The model under review builds one solid part; all positions refer to its coordinate system, in mm. Face numbers are marked on the shaded views. A direction names the side the tool comes from. Round coordinates to 2 decimals unless told otherwise and drop trailing zeros. Order: outer loops, then holes, each group sorted by start corner. A loop starts at its lowest first (then second) coordinate and runs counter-clockwise, first axis right, second up. Notation, with made-up numbers: M -18,82.25 L 30,82.25 A22 ccw 30,97.25 Z; hole C 62.5,61.25 d7. An arc over 180 degrees is marked long. Answer as a JSON object with one key per item and string values. Group by question number.
1) For the marked faces 4 and 5, list the 3-axis set-ups (+Z, -Z, +X, -X, +Y, -Y) from which the entire face can be reached by the end or side of a thin tool; tool diameter is ignored.
2) Consider section A-A, the plane x = 0. Write out the cut boundary in (y, z), then the cut area to 3 significant figures.
3) Insertion check: pin 1 Ø8 at (y, z) = (-14, 21.5) entering from +X; pin 2 Ø7 at (x, z) = (15, 30) entering from -Y; pin 3 Ø10 at (y, z) = (-11.5, 22.5) entering from +X; pin 4 Ø8 at (y, z) = (-3.5, 21.5) entering from -X. Each pin has a flat end and moves straight along its axis. Give the tip position at first contact, or say it passes through.
4) To check wall thickness, follow line 1 (Y direction, x = 5.5, z = 11); line 2 (X direction, y = -3.5, z = -4.5); line 3 (X direction, y = -1.25, z = -5). State the ranges of each line that lie inside material, in increasing order.
5) Consider section D-D, the plane z = 33. Write out the cut boundary in (x, y).
6) Consider section C-C, the plane z = 5. Write out the cut boundary in (x, y), then the cut area to 3 significant figures.
7) Consider section B-B, the plane y = -4.25. Write out the cut boundary in (x, z).
8) The part is to be moulded in two halves that separate along Z. For the marked faces 1, 2 and 3, say which applies: +Z half, -Z half, draft (parallel to the pull), parting line (faces both ways), or undercut.
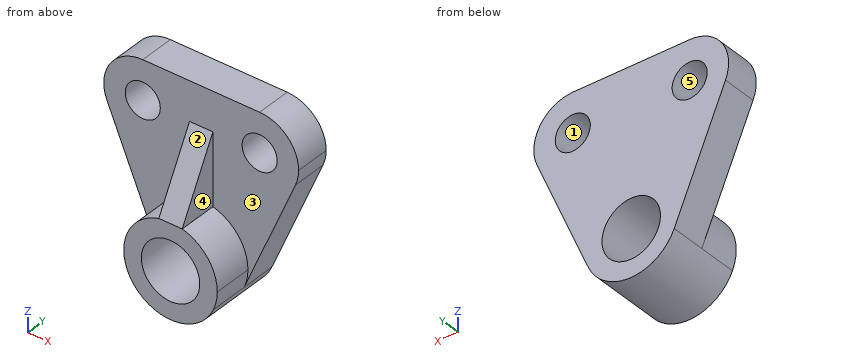
```python
from build123d import *

# Parameters (mm, degrees)
F0_R     = 4.5
F1_DEPTH = 9
F2_DEPTH = 19
F0_R_2   = 7.5
F4_DEPTH = 19
F5_DEPTH = 28.001


with BuildPart() as f1:
    # F0 (on Front) → F1 (new body)
    with BuildSketch(Plane.XZ):
        with BuildLine():
            ThreePointArc((-3, 11.61895), (0, 12), (3, 11.61895))
            Line((3, 11.61895), (3, 30))
            Line((3, 30), (-3, 30))
            Line((-3, 30), (-3, 11.61895))
        make_face()
        with BuildLine():
            ThreePointArc((3, 11.61895), (9.486833, 7.348469), (12, 0))
            ThreePointArc((12, 0), (11.756027, -2.407453), (11.034028, -4.717014))
            Line((11.034028, -4.717014), (24.195023, 26.069155))
            ThreePointArc((24.195023, 26.069155), (6.654089, 24.4913), (15, 40))
            Line((15, 40), (-15, 40))
            ThreePointArc((-15, 40), (-7.928932, 37.071068), (-5, 30))
            ThreePointArc((-5, 30), (-12.993789, 20.203311), (-24.195023, 26.069155))
            Line((-24.195023, 26.069155), (-11.034028, -4.717014))
            ThreePointArc((-11.034028, -4.717014), (-10.768213, 5.295808), (-3, 11.61895))
            Line((-3, 11.61895), (-3, 30))
            Line((-3, 30), (3, 30))
            Line((3, 30), (3, 11.61895))
        make_face()
        with BuildLine():
            ThreePointArc((-15, 40), (-23.345911, 35.5087), (-24.195023, 26.069155))
            ThreePointArc((-24.195023, 26.069155), (-12.993789, 20.203311), (-5, 30))
            ThreePointArc((-5, 30), (-7.928932, 37.071068), (-15, 40))
        make_face()
        with Locations((-15, 30)):
            Circle(F0_R, mode=Mode.SUBTRACT)
        with BuildLine():
            ThreePointArc((15, 40), (6.654089, 24.4913), (24.195023, 26.069155))
            ThreePointArc((24.195023, 26.069155), (24.796689, 27.993789), (25, 30))
            ThreePointArc((25, 30), (22.071068, 37.071068), (15, 40))
        make_face()
        with Locations((15, 30)):
            Circle(F0_R, mode=Mode.SUBTRACT)
    extrude(amount=F1_DEPTH)

    # F0 (on Front) → F2 (join)
    with BuildSketch(Plane.XZ):
        with BuildLine():
            ThreePointArc((-3, 11.61895), (0, 12), (3, 11.61895))
            Line((3, 11.61895), (3, 30))
            Line((3, 30), (-3, 30))
            Line((-3, 30), (-3, 11.61895))
        make_face()
    extrude(amount=F2_DEPTH)

    # F0 (on Front) → F4 (join)
    with BuildSketch(Plane.XZ):
        with BuildLine():
            ThreePointArc((11.034028, -4.717014), (11.756027, -2.407453), (12, 0))
            ThreePointArc((12, 0), (9.486833, 7.348469), (3, 11.61895))
            ThreePointArc((3, 11.61895), (0, 12), (-3, 11.61895))
            ThreePointArc((-3, 11.61895), (-10.768213, 5.295808), (-11.034028, -4.717014))
            ThreePointArc((-11.034028, -4.717014), (0, -12), (11.034028, -4.717014))
        make_face()
        Circle(F0_R_2, mode=Mode.SUBTRACT)
    extrude(amount=F4_DEPTH)

    # F3 (on face) → F5 (cut, through all)
    with BuildSketch(Plane(origin=(-3, 0, 0), x_dir=(0, -1, 0), z_dir=(-1, 0, 0))):
        Polygon((19, 30), (9, 30), (19, 11.61895), align=None)
    extrude(amount=-F5_DEPTH, mode=Mode.SUBTRACT)


solid = f1.part
```
Results list:
{
 "1": {"face 4": "+Z, +X, -Y", "face 5": "+Y, -Y"},
 "2": {"outline": "M -19,-12 L 0,-12 L 0,-7.5 L -19,-7.5 Z; M -19,7.5 L 0,7.5 L 0,40 L -9,40 L -9,30 L -19,11.62 Z", "area": "511 mm^2"},
 "3": {"pin 1": "x = 3", "pin 2": "through", "pin 3": "x = 24.48", "pin 4": "x = -23.95"},
 "4": {"line 1": "-9 to 0", "line 2": "-11.13 to -6, 6 to 11.13", "line 3": "-10.91 to -5.59, 5.59 to 10.91"},
 "5": {"outline": "M -24.54,-9 L -18.35,-9 L -18.35,0 L -24.54,0 Z; M -11.65,-9 L 11.65,-9 L 11.65,0 L -11.65,0 Z; M 18.35,-9 L 24.54,-9 L 24.54,0 L 18.35,0 Z"},
 "6": {"outline": "M -15.19,-9 L -10.91,-9 L -10.91,-19 L -5.59,-19 L -5.59,0 L -15.19,0 Z; M 5.59,-19 L 10.91,-19 L 10.91,-9 L 15.19,-9 L 15.19,0 L 5.59,0 Z", "area": "279 mm^2"},
 "7": {"outline": "M -24.2,26.07 L -11.03,-4.72 A12 ccw 11.03,-4.72 L 24.2,26.07 A10 ccw 25,30 A10 ccw 15,40 L -15,40 A10 ccw Z; hole C -15,30 d9; hole C 0,0 d15; hole C 15,30 d9"},
 "8": {"face 1": "undercut", "face 2": "+Z half", "face 3": "draft"}
}
